```python
from build123d import *

# Parameters (mm, degrees)
F1_DEPTH    = 20
F2_T1_DEPTH = 29.6148139682
F2_T3_DEPTH = 30.8021727026


# Not quite as in the source:
# - a fillet or chamfer that OpenCascade refuses, or shapes differently, is made with other operations: its cross-section is extruded or revolved along the edge and cut away or added


with BuildPart() as f1:
    # F0 (on Top) → F1 (new body)
    with BuildSketch(Plane.XY):
        with BuildLine():
            ThreePointArc((15.9085457216, 17.9699241241), (21.8838421823, 9.8538039021), (24, 0))
            ThreePointArc((24, 0), (-10.4300926413, -21.6151143299), (-14.9344306245, 18.7873037427))
            Line((-14.9344306245, 18.7873037427), (-16.9256880412, 21.2922775751))
            ThreePointArc((-16.9256880411, 21.2922775751), (-11.8207716601, -24.4971295739), (27.2, 0))
            ThreePointArc((27.2, 0), (24.8016878066, 11.1676444224), (18.0296851511, 20.3659140073))
            Line((18.0296851511, 20.3659140073), (15.9085457216, 17.9699241241))
        make_face()
    extrude(amount=F1_DEPTH)

    # F2: fillet of radius 2 on 4 edges, made by hand

    # F2_s2 → F2_t1 (cut)
    with BuildSketch(Plane.XY.offset(-4.8074069841)):
        with BuildLine():
            ThreePointArc((-16.3353575734, 17.5828351795), (-15.7022990684, 18.8976894845), (-16.131028726, 20.2926073298))
            Line((-16.131028726, 20.2926073298), (-14.9344306245, 18.7873037427))
            ThreePointArc((-14.9344306245, 18.7873037427), (-15.6464884117, 18.1985548982), (-16.3353575734, 17.5828351795))
        make_face()
        with BuildLine():
            ThreePointArc((17.2437110419, 16.6929455011), (16.6811829734, 18.0394844298), (17.183193285, 19.4097364364))
            Line((17.183193285, 19.4097364364), (15.9085457216, 17.9699241241))
            ThreePointArc((15.9085457216, 17.9699241241), (16.5884206822, 17.3442872229), (17.2437110419, 16.6929455011))
        make_face()
    extrude(amount=F2_T1_DEPTH, mode=Mode.SUBTRACT)

    # F2_s4 → F2_t3 (cut)
    with BuildSketch(Plane.XY.offset(-5.4010863513)):
        with BuildLine():
            ThreePointArc((-18.5621612385, 19.8818050024), (-17.0493571531, 20.4144285626), (-15.6316877963, 19.6644434612))
            Line((-15.6316877963, 19.6644434612), (-16.9256880412, 21.2922775751))
            ThreePointArc((-16.9256880412, 21.2922775751), (-17.7579339971, 20.6032953713), (-18.5621612385, 19.8818050024))
        make_face()
        with BuildLine():
            ThreePointArc((19.5891550007, 18.8707447219), (18.1066850122, 19.482747002), (16.6512822795, 18.8089021064))
            Line((16.6512822795, 18.8089021064), (18.0296851511, 20.3659140073))
            ThreePointArc((18.0296851511, 20.3659140073), (18.8242706735, 19.6338186202), (19.5891550007, 18.8707447219))
        make_face()
    extrude(amount=F2_T3_DEPTH, mode=Mode.SUBTRACT)


solid = f1.part
```
Input: part model. Units: mm. Frame: model coordinates. Round coordinates to 2 decimals unless told otherwise and drop trailing zeros. Loops run counter-clockwise (first coordinate to the right, second up) from the corner with the lowest first, then second, coordinate; pieces in that order, holes last. Notation, with made-up numbers: (62, 26.25) -> (85, 26.25) arc R26 cw to (85, 41.25) -> close; hole circle Ø4 at (55, 67). An arc over 180 degrees is marked (long way). One line per item, written item: value.
(1) Material intervals for line 1 (X direction, y = 0, z = 12); line 2 (X direction, y = 2.5, z = 14.75); line 3 (Y direction, x = -16, z = 9.75), sorted ascending. Write a range as [from, to].
Geometry check:
line 1: [-27.2, -24], [24, 27.2]
line 2: [-27.08, -23.87], [23.87, 27.08]
line 3: [-22, -17.89], [17.99, 20.02]
(2) Section B-B (z = 14.75). Return the cut outline in (x, y).
Geometry check:
outline: (-18.56, 19.88) arc R27.2 ccw (long way) to (19.59, 18.87) arc R2 ccw to (16.95, 19.08) arc R2 ccw to (17.24, 16.69) arc R24 cw (long way) to (-16.34, 17.58) arc R2 ccw to (-15.91, 19.95) arc R2 ccw to start
(3) Section D-D (x = 0). Return the cut outline in (y, z).
Geometry check:
outline: (-27.2, 0) -> (-24, 0) -> (-24, 20) -> (-27.2, 20) -> close
(4) Pin query (flat end, axial travel): pin 1 (4 mm diameter, centred on x = 14.5, z = 10.5, fed in from +Y); pin 2 (1.5 mm diameter, centred on y = 13.5, z = 3.5, fed in from -X); pin 3 (10 mm diameter, centred on x = -2.5, z = 3.5, fed in from +Y); pin 4 (10 mm diameter, centred on x = 12, y = -10.5, fed in from +Z). Return the tip coordinate at first contact, or that it passes through.
Geometry check:
pin 1: y = -17.43
pin 2: x = -24.03
pin 3: y = -22.8
pin 4: through
(5) Mould query, pull axis Y, two halves, no side actions, for faces 1 (the face through (-15.73, 18.68, 9.86)), 2 (the face through (16.7, 17.8, 9.9)), 3 (the face through (-8, -23, 20)), 4 (the face through (18.329, 19.475, 9.86)). Classes: pulls with the +Y half, pulls with the -Y half, needs draft (parallel to the pull), parting line crosses it, or undercut.
Geometry check:
face 1: undercut
face 2: undercut
face 3: needs draft
face 4: pulls with the +Y half
(6) Section A-A (y = 12.5). Return the cut outline in (x, z).
Geometry check:
outline: (-24.16, 0) -> (-20.49, 0) -> (-20.49, 20) -> (-24.16, 20) -> close; (20.49, 0) -> (24.16, 0) -> (24.16, 20) -> (20.49, 20) -> close
(7) Section C-C (x = -22.5). Return the cut outline in (y, z), plus the area to 3 significant figures.
Geometry check:
outline: (-15.28, 0) -> (-8.35, 0) -> (-8.35, 20) -> (-15.28, 20) -> close; (8.35, 0) -> (15.28, 0) -> (15.28, 20) -> (8.35, 20) -> close
area: 277 mm2
